Read the model definition and answer for the solid it produces. Units are mm, in the model's axes. A direction names the side the tool comes from. Give positions to 0.01 mm unless a question says otherwise; leave off trailing zeros. Write each loop counter-clockwise with the first axis right and the second up, starting at its lowest first coordinate (ties: lowest second). Pieces come first, ordered by that corner, then holes. Notation, with made-up numbers: M -36.5,89 L -19.5,89 A12 cw -19.5,100 Z; hole C 68.5,-21 d8. An arc over 180 degrees is marked long. Answer as CSV lines item,"result". Start each with the question number.
```python
from build123d import *

# Parameters (mm, degrees)
F1_DEPTH = 10
F2_R     = 6
F2_R_2   = 2
F3_DEPTH = 25
F4_R     = 3
F5_DEPTH = 24.5


with BuildPart() as f1:
    # F0 (on Top) → F1 (new body)
    with BuildSketch(Plane.XY):
        Polygon((-60, -40), (-60, -65), (60, -65), (60, -40), (50, -40), (40, 0), (-40, 0), (-50, -40), align=None)
    extrude(amount=F1_DEPTH)

    # F2 (on Top) → F3 (cut)
    with BuildSketch(Plane.XY):
        with Locations((-15, -26)):
            Circle(F2_R)
        with Locations((-30.5, -10.5)):
            Circle(F2_R_2)
        with Locations((0.5, -10.5)):
            Circle(F2_R_2)
        with Locations((-30.5, -41.5)):
            Circle(F2_R_2)
        with Locations((0.5, -41.5)):
            Circle(F2_R_2)
    extrude(amount=F3_DEPTH, mode=Mode.SUBTRACT)

    # F4 (on Top) → F5 (cut)
    with BuildSketch(Plane.XY):
        with Locations((-45, -50)):
            Circle(F4_R)
        with Locations((-15, -50)):
            Circle(F4_R)
        with Locations((45, -50)):
            Circle(F4_R)
        with Locations((15, -50)):
            Circle(F4_R)
    extrude(amount=F5_DEPTH, mode=Mode.SUBTRACT)


solid = f1.part
```
1. Find section B-B on x = -15. Determine the outline of the cut face in (y, z).
2. Given pin 1 (3 mm diameter, centred on x = 55.5, z = 7.5, fed in from +Y); pin 2 (4 mm diameter, centred on y = -26, z = 7.5, fed in from -X); pin 3 (3.5 mm diameter, centred on x = 15, y = -50, fed in from +Z); pin 4 (1.5 mm diameter, centred on x = 17.5, z = 6, fed in from +Y), each flat-ended and moving along its own axis, determine where each tip first touches the part or whether it passes through.
3. Determine the mould class of faces 1 (the face through (-1, -32, 10)), 2 (the face through (-45, -47, 5)), 3 (the face through (45, -20, 5)) for opening direction X: +X half, -X half, draft (parallel to the pull), parting line (faces both ways), or undercut.
4. Find section A-A on y = -26. Determine the outline of the cut face in (x, z), then the cut area to 3 significant figures.
5. Find section C-C on z = 8.25. State how many separate pieces and enclosed holes the cut face has, then the cut area to 3 significant figures.
6. For faces 4 (the face through (55, -40, 5)), 5 (the face through (-55, -40, 5)), 6 (the face through (-1, -32, 0)), determine the directions among +Z, -Z, +X, -X, +Y, -Y from which every point of the face is accessible in a straight line to the end or side of a thin tool.
7. Find section D-D on y = -50. Determine the outline of the cut face in (x, z), then the cut area to 3 significant figures.
8. Find the intervals of material crossed by line 1 (X direction, y = -50, z = 5); line 2 (Y direction, x = -15, z = 9.75); line 3 (X direction, y = -10.5, z = 6) (3 decimals), in increasing order. Write a range as [from, to].
Computed:
1,outline,"M -65,0 L -53,0 L -53,10 L -65,10 Z; M -47,0 L -32,0 L -32,10 L -47,10 Z; M -20,0 L 0,0 L 0,10 L -20,10 Z"
2,pin 1,"stops at y = -40"
2,pin 2,"stops at x = -47"
2,pin 3,"passes through"
2,pin 4,"stops at y = 0"
3,face 1,"draft"
3,face 2,"undercut"
3,face 3,"+X half"
4,outline,"M -46.5,0 L -21,0 L -21,10 L -46.5,10 Z; M -9,0 L 46.5,0 L 46.5,10 L -9,10 Z"
4,area,"810 mm^2"
5,separate pieces,"1"
5,enclosed holes,"9"
5,area,"6,320 mm^2"
6,face 4,"+Z, -Z, +X, +Y"
6,face 5,"+Z, -Z, -X, +Y"
6,face 6,"-Z, +X, -X, +Y, -Y"
7,outline,"M -60,0 L -48,0 L -48,10 L -60,10 Z; M -42,0 L -18,0 L -18,10 L -42,10 Z; M -12,0 L 12,0 L 12,10 L -12,10 Z; M 18,0 L 42,0 L 42,10 L 18,10 Z; M 48,0 L 60,0 L 60,10 L 48,10 Z"
7,area,"960 mm^2"
8,line 1,"x = [-60, -48], [-42, -18], [-12, 12], [18, 42], [48, 60]"
8,line 2,"y = [-65, -53], [-47, -32], [-20, 0]"
8,line 3,"x = [-42.625, -32.5], [-28.5, -1.5], [2.5, 42.625]"
